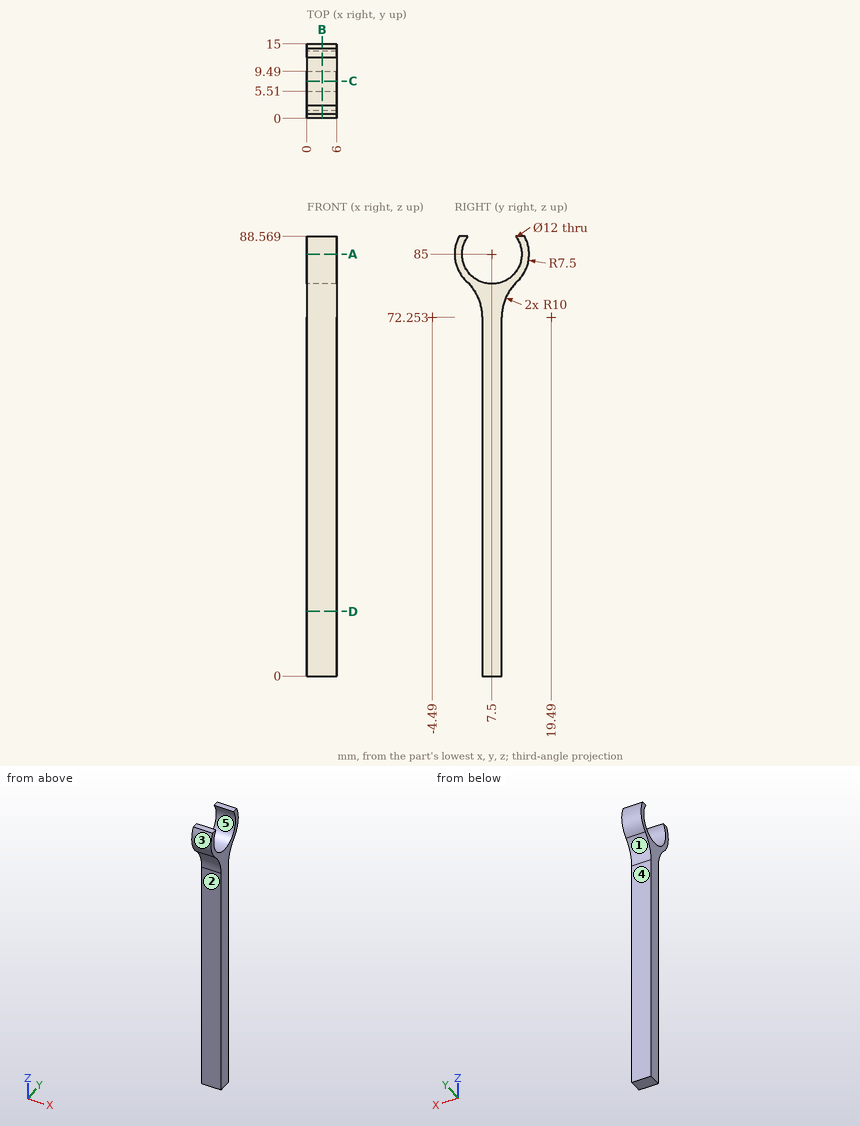
Geometry: see drawing. Coordinates: mm, zero at the bounding-box minimum. A direction names the side the tool comes from. Round coordinates to 2 decimals unless told otherwise and drop trailing zeros. Write each loop counter-clockwise with the first axis right and the second up, starting at its lowest first coordinate (ties: lowest second). Pieces come first, ordered by that corner, then holes.
Item 1: Section query A-A (z = 85). Return loops of the section in (x, y), plus the area to 3 significant figures.
Item 2: Pin query (flat end, axial travel): P1, Ø1, axis at y = 7.5, z = 48, coming from the -X side; P2, Ø1.5, axis at x = 1, y = 6, coming from the +Z side; P3, Ø2, axis at x = 4.5, y = 7.5, coming from the +Z side; P4, Ø3, axis at x = 4.5, z = 21.5, coming from the +Y side. Return the tip coordinate at first contact, or that it passes through.
Item 3: Section query D-D (z = 13). Return loops of the section in (x, y).
Item 4: Mould query, pull axis Y, two halves, no side actions, for the marked faces 3, 4 and 5. Classes: +Y half, -Y half, draft (parallel to the pull), parting line (faces both ways), or undercut.
Item 5: Material intervals for L1, parallel to Y at x = 1.3, z = 85; L2, parallel to Z at x = 4.2, y = 7.5; L3, parallel to Y at x = 4.35, z = 30.5, sorted ascending.
Item 6: Set-up query: the marked faces 1 and 2. Return all of +Z, -Z, +X, -X, +Y, -Y with unobstructed straight access to the full face (end or side cutting, diameter ignored); none if empty.
Item 7: Section query C-C (y = 7.5). Return loops of the section in (x, z).
Item 8: Section query B-B (x = 3.05). Return loops of the section in (y, z).
Completed:
1. outline: (0, 0) - (6, 0) - (6, 1.5) - (0, 1.5) - close; (0, 13.5) - (6, 13.5) - (6, 15) - (0, 15) - close
1. area: 18.0 mm2
2. P1: stops at x = 0
2. P2: stops at z = 79.44
2. P3: stops at z = 79.08
2. P4: stops at y = 9.49
3. outline: (0, 5.51) - (6, 5.51) - (6, 9.49) - (0, 9.49) - close
4. face 3: -Y half
4. face 4: +Y half
4. face 5: undercut
5. L1: y = 0 to 1.5, 13.5 to 15
5. L2: z = 0 to 79
5. L3: y = 5.51 to 9.49
6. face 1: -Z, +X, -X, +Y
6. face 2: -Z, +X, -X, -Y
7. outline: (0, 0) - (6, 0) - (6, 79) - (0, 79) - close
8. outline: (0.9, 88.57) arc R7.5 ccw to (2.36, 79.54) arc R10 cw to (5.51, 72.25) - (5.51, 0) - (9.49, 0) - (9.49, 72.25) arc R10 cw to (12.64, 79.54) arc R7.5 ccw to (14.1, 88.57) - (12.32, 88.57) arc R6 cw (long way) to (2.68, 88.57) - close
